The listing builds one solid part. Answer for the finished solid, in the listing's coordinates (mm). Face numbers are marked on the shaded views. Give positions to 0.01 mm unless a question says otherwise; leave off trailing zeros. Use a Markdown table: item, result. Add a question column.
1) Straight lines are drawn through the part: line 1 (Z direction, x = -88, y = 212); line 2 (X direction, y = 166, z = 4). For each, find the intervals that lie inside material, in ascending order.
2) Flat-ended cylindrical pins translate along their axes: pin 1 (6.5 mm diameter, centred on x = 65.09, y = 164.13, fed in from -Z); pin 2 (2.5 mm diameter, centred on x = -51, z = 6.5, fed in from +Y). Find the tip coordinate at first contact, or state that the pin passes through.
3) The mould has two halves that part along Z. Classify the marked faces 1 and 2: released by +Z, released by -Z, zero draft, split by the parting line, or undercut.
from build123d import *

# Parameters (mm, degrees)
F0_W     = 203.2
F0_H     = 431.8
F0_R     = 2.54
F1_DEPTH = 12.7
F2_R     = 2.54
F3_DEPTH = 12.701
F4_R     = 2.54
F5_DEPTH = 12.7
F6_R     = 2.3114
F7_DEPTH = 25.4
F8_DEPTH = 25.4


with BuildPart() as f1:
    # F0 (on Top) → F1 (new body)
    with BuildSketch(Plane.XY):
        Rectangle(F0_W, F0_H)
        with Locations((-65.0875, -195.834)):
            Circle(F0_R, mode=Mode.SUBTRACT)
        with Locations((-65.0875, -135.8392)):
            Circle(F0_R, mode=Mode.SUBTRACT)
        with Locations((-65.0875, -75.8444)):
            Circle(F0_R, mode=Mode.SUBTRACT)
        with Locations((-65.0875, -15.8496)):
            Circle(F0_R, mode=Mode.SUBTRACT)
        with Locations((65.0875, -195.834)):
            Circle(F0_R, mode=Mode.SUBTRACT)
        with Locations((65.0875, -135.8392)):
            Circle(F0_R, mode=Mode.SUBTRACT)
        with Locations((65.0875, -75.8444)):
            Circle(F0_R, mode=Mode.SUBTRACT)
        with Locations((65.0875, -15.8496)):
            Circle(F0_R, mode=Mode.SUBTRACT)
        with Locations((-65.0875, 44.1452)):
            Circle(F0_R, mode=Mode.SUBTRACT)
        with Locations((-65.0875, 104.14)):
            Circle(F0_R, mode=Mode.SUBTRACT)
        with Locations((-65.0875, 164.1348)):
            Circle(F0_R, mode=Mode.SUBTRACT)
        with Locations((65.0875, 44.1452)):
            Circle(F0_R, mode=Mode.SUBTRACT)
        with Locations((65.0875, 104.14)):
            Circle(F0_R, mode=Mode.SUBTRACT)
        with Locations((65.0875, 164.1348)):
            Circle(F0_R, mode=Mode.SUBTRACT)
    extrude(amount=F1_DEPTH)

    # F2 (on face) → F3 (cut, through all)
    with BuildSketch(Plane.XY.offset(12.7)):
        with Locations((-22.86, 192.0494)):
            Circle(F2_R)
        with Locations((-22.86, 205.0796)):
            Circle(F2_R)
        with Locations((23.1394, 205.0796)):
            Circle(F2_R)
        with Locations((23.1394, 192.0494)):
            Circle(F2_R)
        with Locations((-22.86, -205.867)):
            Circle(F2_R)
        with Locations((23.1394, -205.867)):
            Circle(F2_R)
    extrude(amount=-F3_DEPTH, mode=Mode.SUBTRACT)

    # F4 (on face) → F5 (cut)
    with BuildSketch(Plane(origin=(0, 215.9, 0), x_dir=(-1, 0, 0), z_dir=(0, 1, 0))):
        with Locations((-88.9, 6.35)):
            Circle(F4_R)
        with Locations((-50.8, 6.35)):
            Circle(F4_R)
        with Locations((50.8, 6.35)):
            Circle(F4_R)
        with Locations((88.9, 6.35)):
            Circle(F4_R)
        with Locations((12.7, 6.35)):
            Circle(F4_R)
        with Locations((-12.7, 6.35)):
            Circle(F4_R)
    extrude(amount=-F5_DEPTH, mode=Mode.SUBTRACT)

    # F6 (on face) → F7 (cut)
    with BuildSketch(Plane.XY.offset(12.7)):
        with Locations((-75.4888, -59.451528)):
            Circle(F6_R)
        with Locations((-75.4888, -85.740528)):
            Circle(F6_R)
        with Locations((-75.4888, -112.029528)):
            Circle(F6_R)
        with Locations((75.4888, -59.451528)):
            Circle(F6_R)
        with Locations((75.4888, -85.740528)):
            Circle(F6_R)
        with Locations((75.4888, -112.029528)):
            Circle(F6_R)
    extrude(amount=-F7_DEPTH, mode=Mode.SUBTRACT)

    # F6 (on face) → F8 (cut)
    with BuildSketch(Plane.XY.offset(12.7)):
        with Locations((-75.4888, -59.451528)):
            Circle(F6_R)
        with Locations((-75.4888, -85.740528)):
            Circle(F6_R)
        with Locations((-75.4888, -112.029528)):
            Circle(F6_R)
        with Locations((75.4888, -59.451528)):
            Circle(F6_R)
        with Locations((75.4888, -85.740528)):
            Circle(F6_R)
        with Locations((75.4888, -112.029528)):
            Circle(F6_R)
    extrude(amount=-F8_DEPTH, mode=Mode.SUBTRACT)


solid = f1.part
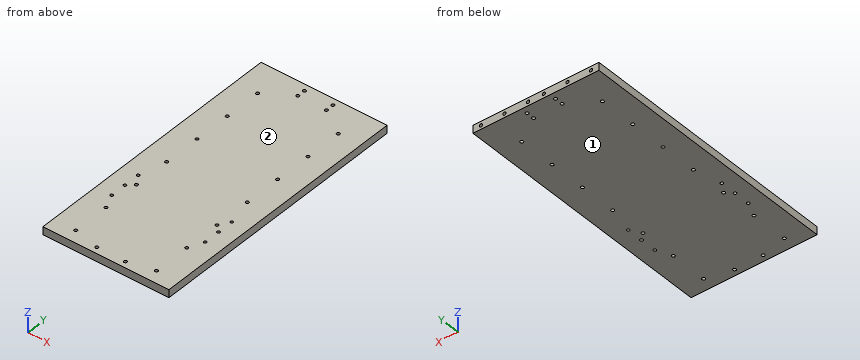
The answers:
| question | item | result |
|---|---|---|
| 1 | line 1 | 0 to 3.97, 8.73 to 12.7 |
| 1 | line 2 | -101.6 to -66.81, -63.36 to 63.36, 66.81 to 101.6 |
| 2 | pin 1 | z = 0 |
| 2 | pin 2 | y = 203.2 |
| 3 | face 1 | released by -Z |
| 3 | face 2 | released by +Z |
